from build123d import *

# Parameters (mm, degrees)
BOSS_EXTRUDE1_DEPTH    = 6.35
F_10_32_TAPPED_HOLE1_D = 4.0386
F_10_CLEARANCE_HOLE1_D = 5.1054
SKETCH6_W              = 25.4
SKETCH6_H              = 5.08
CUT_EXTRUDE1_DEPTH     = 2.54
CHAMFER1_SIZE          = 2.54
CUT_EXTRUDE2_DEPTH     = 7.35


with BuildPart() as part:
    # Sketch1 → Boss-Extrude1 (new body)
    with BuildSketch(Plane(origin=(0, 0, 0), x_dir=(0, 0, -1), z_dir=(1, 0, 0))):
        with BuildLine():
            Line((0, 0), (127, 0))
            Line((127, 0), (127, 25.4))
            Line((127, 25.4), (41.275, 25.4))
            ThreePointArc((41.275, 25.4), (39.02993597, 26.32993597), (38.1, 28.575))
            Line((38.1, 28.575), (38.1, 44.45))
            Line((38.1, 44.45), (30.1625, 44.45))
            Line((30.1625, 44.45), (30.1625, 27.178))
            ThreePointArc((30.1625, 27.178), (29.641735857, 25.920764143), (28.3845, 25.4))
            Line((28.3845, 25.4), (22.4155, 25.4))
            ThreePointArc((22.4155, 25.4), (21.158264143, 25.920764143), (20.6375, 27.178))
            Line((20.6375, 27.178), (20.6375, 44.45))
            Line((20.6375, 44.45), (12.7, 44.45))
            Line((12.7, 44.45), (12.7, 28.575))
            ThreePointArc((12.7, 28.575), (11.77006403, 26.32993597), (9.525, 25.4))
            Line((9.525, 25.4), (0, 25.4))
            Line((0, 25.4), (0, 0))
        make_face()
    extrude(amount=BOSS_EXTRUDE1_DEPTH)

    # #10-32 Tapped Hole1 (through all)
    with Locations(Plane(origin=(6.35, 0, 0), x_dir=(0, 0, -1), z_dir=(1, 0, 0))):
        with Locations((12.7, 12.7), (25.4, 12.7), (38.1, 12.7)):
            Hole(F_10_32_TAPPED_HOLE1_D / 2)

    # #10 Clearance Hole1 (through all)
    with Locations(Plane(origin=(6.35, 0, 0), x_dir=(0, 0, -1), z_dir=(1, 0, 0))):
        with Locations((119.0625, 17.4625), (109.5375, 7.9375), (34.13125, 31.75), (16.66875, 31.75)):
            Hole(F_10_CLEARANCE_HOLE1_D / 2)

    # Sketch6 → Cut-Extrude1 (cut)
    with BuildSketch(Plane(origin=(6.35, 0, 0), x_dir=(0, 0, -1), z_dir=(1, 0, 0))):
        with Locations((25.4, 38.1)):
            Rectangle(SKETCH6_W, SKETCH6_H)
    extrude(amount=-CUT_EXTRUDE1_DEPTH, mode=Mode.SUBTRACT)

    # Chamfer1
    chamfer1_edges = [part.edges().sort_by_distance(p)[0] for p in [
        (3.175, 25.4, 0),
        (3.175, 44.45, -12.7),
        (3.175, 44.45, -38.1),
        (3.175, 25.4, -127),
        (3.175, 0, -127),
        (3.175, 0, 0),
    ]]
    chamfer(chamfer1_edges, length=CHAMFER1_SIZE)

    # Sketch7 → Cut-Extrude2 (cut, through all)
    with BuildSketch(Plane(origin=(6.35, 0, 0), x_dir=(0, 0, -1), z_dir=(1, 0, 0))):
        with BuildLine():
            Line((60.325, 19.05), (92.075, 19.05))
            ThreePointArc((92.075, 19.05), (98.425, 12.7), (92.075, 6.35))
            Line((92.075, 6.35), (60.325, 6.35))
            ThreePointArc((60.325, 6.35), (53.975, 12.7), (60.325, 19.05))
        make_face()
    extrude(amount=-CUT_EXTRUDE2_DEPTH, mode=Mode.SUBTRACT)


solid = part.part
Work out the finished part from the listing and answer in its coordinate system (mm). A direction names the side the tool comes from. Coordinates: 2 decimals unless noted, no trailing zeros. Order: outer loops, then holes, each group sorted by start corner. A loop starts at its lowest first (then second) coordinate and runs counter-clockwise, first axis right, second up. Notation, with made-up numbers: (-29.75, 60.5) - (-0.75, 60.5) arc R24 ccw to (-0.75, 95.5) - close; hole circle Ø11 at (68.5, -1). An arc over 180 degrees is marked (long way). Put each result on its own line as item: value. Start each with the question number.
1) Find section D-D (x = 1.75). State how many separate pieces and enclosed holes the cut face has, plus the area to 3 significant figures.
2) For a pull along Y with two mould halves and no side action, classify faces 1 (the flat face through (3.81, 38, -17)), 2 (the flat face through (3, 0, -63)), 3 (the flat face through (6.35, 43, -34)), 4 (the flat face through (3, 25.4, -83)) as released by +Y, released by -Y, zero draft, split by the parting line, or undercut.
3) Flat-ended cylindrical pins translate along their axes: pin 1 (3 mm diameter, centred on x = 4.5, z = -26, fed in from +Y); pin 2 (4 mm diameter, centred on y = 38.5, z = -17, fed in from +X); pin 3 (1.9 mm diameter, centred on x = 3.5, y = 37.5, fed in from +Z). Find the tip coordinate at first contact, or state that the pin passes through.
4) Find the intervals of material crossed by line 1 (Y direction, x = 5.5, z = -81); line 2 (Z direction, x = 0.5, y = 14.5), in increasing order. Write a range as from..to.
5) For faces 5 (the flat face through (5, 40.64, -34)), 6 (the flat face through (3, 25.4, -6)), 7 (the cylindrical face through (3.219, 12.56, -53.977)), determine the directions among +Z, -Z, +X, -X, +Y, -Y from which every point of the face is accessible in a straight line to the end or side of a thin tool.
6) Find section C-C (y = 31.75). Give the vertices of the cut face in (x, z).
7) Find section A-A (z = -25.4). Give the vertices of the cut face in (x, y).
8) Find section B-B (y = 12.7). Give the vertices of the cut face in (x, z) (3 decimals).
Results list:
1. separate pieces: 1
1. enclosed holes: 8
1. area: 2,860 mm^2
2. face 1: undercut
2. face 2: released by -Y
2. face 3: zero draft
2. face 4: released by +Y
3. pin 1: stops at y = 25.4
3. pin 2: stops at x = 3.81
3. pin 3: stops at z = -12.7
4. line 1: y = 0..6.35, 19.05..25.4
4. line 2: z = -127..-98.16, -54.24..-39.02, -37.18..-26.32, -24.48..-13.62, -11.78..0
5. face 5: +Z, -Z, +X
5. face 6: +Z, +X, -X, +Y
5. face 7: +X, -X
6. outline: (0, -38.1) - (6.35, -38.1) - (6.35, -36.68) - (0, -36.68) - close; (0, -31.58) - (6.35, -31.58) - (6.35, -30.16) - (0, -30.16) - close; (0, -20.64) - (6.35, -20.64) - (6.35, -19.22) - (0, -19.22) - close; (0, -14.12) - (6.35, -14.12) - (6.35, -12.7) - (0, -12.7) - close
7. outline: (0, 0) - (6.35, 0) - (6.35, 10.68) - (0, 10.68) - close; (0, 14.72) - (6.35, 14.72) - (6.35, 25.4) - (0, 25.4) - close
8. outline: (0, -127) - (6.35, -127) - (6.35, -98.425) - (0, -98.425) - close; (0, -53.975) - (6.35, -53.975) - (6.35, -40.119) - (0, -40.119) - close; (0, -36.081) - (6.35, -36.081) - (6.35, -27.419) - (0, -27.419) - close; (0, -23.381) - (6.35, -23.381) - (6.35, -14.719) - (0, -14.719) - close; (0, -10.681) - (6.35, -10.681) - (6.35, 0) - (0, 0) - close
